The model under review builds one solid part; all positions refer to its coordinate system, in mm. A direction names the side the tool comes from. Round coordinates to 2 decimals unless told otherwise and drop trailing zeros. Loops run counter-clockwise (first coordinate to the right, second up) from the corner with the lowest first, then second, coordinate; pieces in that order, holes last. Notation, with made-up numbers: (-23.75, 12.5) -> (-13.75, 12.5) arc R22 ccw to (-13.75, 30.5) -> close; hole circle Ø7 at (34.25, 32). An arc over 180 degrees is marked (long way). Return JSON: item names as keys, results as strings. Group by question number.
```python
from build123d import *

# Parameters (mm, degrees)
SKETCH1_W      = 52
SKETCH1_H      = 21.25
EXTRUDE1_DEPTH = 5
SKETCH2_W      = 20
SKETCH2_H      = 5
EXTRUDE2_DEPTH = 86.5
FILLET1_R      = 6.35
SKETCH3_W      = 19.05
SKETCH3_H      = 50.8
EXTRUDE3_DEPTH = 9.525


with BuildPart() as part:
    # Sketch1 → Extrude1 (new body)
    with BuildSketch(Plane.XY):
        with Locations((26, -10.625)):
            Rectangle(SKETCH1_W, SKETCH1_H)
    extrude(amount=EXTRUDE1_DEPTH)

    # Sketch2 → Extrude2 (add)
    with BuildSketch(Plane.XY.offset(5)):
        with Locations((10, -18.75)):
            Rectangle(SKETCH2_W, SKETCH2_H)
    extrude(amount=EXTRUDE2_DEPTH)

    # Fillet1
    fillet1_edges = [part.edges().sort_by_distance(p)[0] for p in [
        (20, -18.75, 5),
    ]]
    fillet(fillet1_edges, radius=FILLET1_R)

    # Sketch3 → Extrude3 (add)
    with BuildSketch(Plane(origin=(0, -16.25, 0), x_dir=(1, 0, 0), z_dir=(0, 1, 0))):
        with Locations((10, -53)):
            Rectangle(SKETCH3_W, SKETCH3_H)
    extrude(amount=EXTRUDE3_DEPTH)


solid = part.part
```
1. Wall thickness on line 1 (Z direction, x = 15.5, y = -13.5); line 2 (Y direction, x = 4, z = 21); line 3 (Z direction, x = 23, y = -7.75): over which ranges is each line inside the solid? List them lowest first.
2. We need section C-C, the plane y = -19.5. Write out the cut boundary in (x, z), then the cut area to 3 significant figures.
3. Draft analysis for pull direction Z (two halves, no side actions). For faces 1 (the face through (26, -10, 5)), 2 (the face through (52, -11, 2)), 3 (the face through (10, -12, 27.6)), 4 (the face through (10, -12, 78.4)), state which applies: pulls with the +Z half, pulls with the -Z half, needs draft (parallel to the pull), parting line crosses it, or undercut.
4. For P1, Ø12, axis at x = 18.5, z = 32, coming from the +Y side (3 decimals); P2, Ø7.5, axis at y = -10, z = 58, coming from the -X side (3 decimals); P3, Ø5, axis at y = -18, z = 52.5, coming from the +X side, all flat-tipped, find the tip position at first contact; note any pin that passes through.
5. We need section D-D, the plane x = 28.5. Write out the cut boundary in (y, z), then the cut area to 3 significant figures.
6. We need section B-B, the plane z = 59. Write out the cut boundary in (x, y) (3 decimals), then the cut area to 3 significant figures.
7. Tool access review of faces 5 (the face through (20, -19, 51)), 6 (the face through (0.475, -12, 53)), 7 (the face through (19.525, -12, 53)), 8 (the face through (10, -6.725, 53)): name each direction out of +Z, -Z, +X, -X, +Y, -Y from which nothing blocks a thin tool from reaching the whole face with its end or side.
8. We need section A-A, the plane y = -13.75. Write out the cut boundary in (x, z) (3 decimals), then the cut area to 3 significant figures.
Check sheet entries:
{
 "1": {"line 1": "z = 0 to 5, 27.6 to 78.4", "line 2": "y = -21.25 to -16.25", "line 3": "z = 0 to 5"},
 "2": {"outline": "(0, 0) -> (52, 0) -> (52, 5) -> (26.35, 5) arc R6.35 cw to (20, 11.35) -> (20, 91.5) -> (0, 91.5) -> close", "area": "2,000 mm²"},
 "3": {"face 1": "undercut", "face 2": "needs draft", "face 3": "undercut", "face 4": "pulls with the +Z half"},
 "4": {"P1": "stops at y = -6.725", "P2": "stops at x = 0.475", "P3": "stops at x = 20"},
 "5": {"outline": "(-21.25, 0) -> (0, 0) -> (0, 5) -> (-21.25, 5) -> close", "area": "106 mm²"},
 "6": {"outline": "(0, -21.25) -> (20, -21.25) -> (20, -16.25) -> (19.525, -16.25) -> (19.525, -6.725) -> (0.475, -6.725) -> (0.475, -16.25) -> (0, -16.25) -> close", "area": "281 mm²"},
 "7": {"face 5": "+Z, +X, +Y, -Y", "face 6": "+Z, -X, +Y", "face 7": "+Z, +X, +Y", "face 8": "+Z, +X, -X, +Y"},
 "8": {"outline": "(0, 0) -> (52, 0) -> (52, 5) -> (0, 5) -> close; (0.475, 27.6) -> (19.525, 27.6) -> (19.525, 78.4) -> (0.475, 78.4) -> close", "area": "1,230 mm²"}
}
